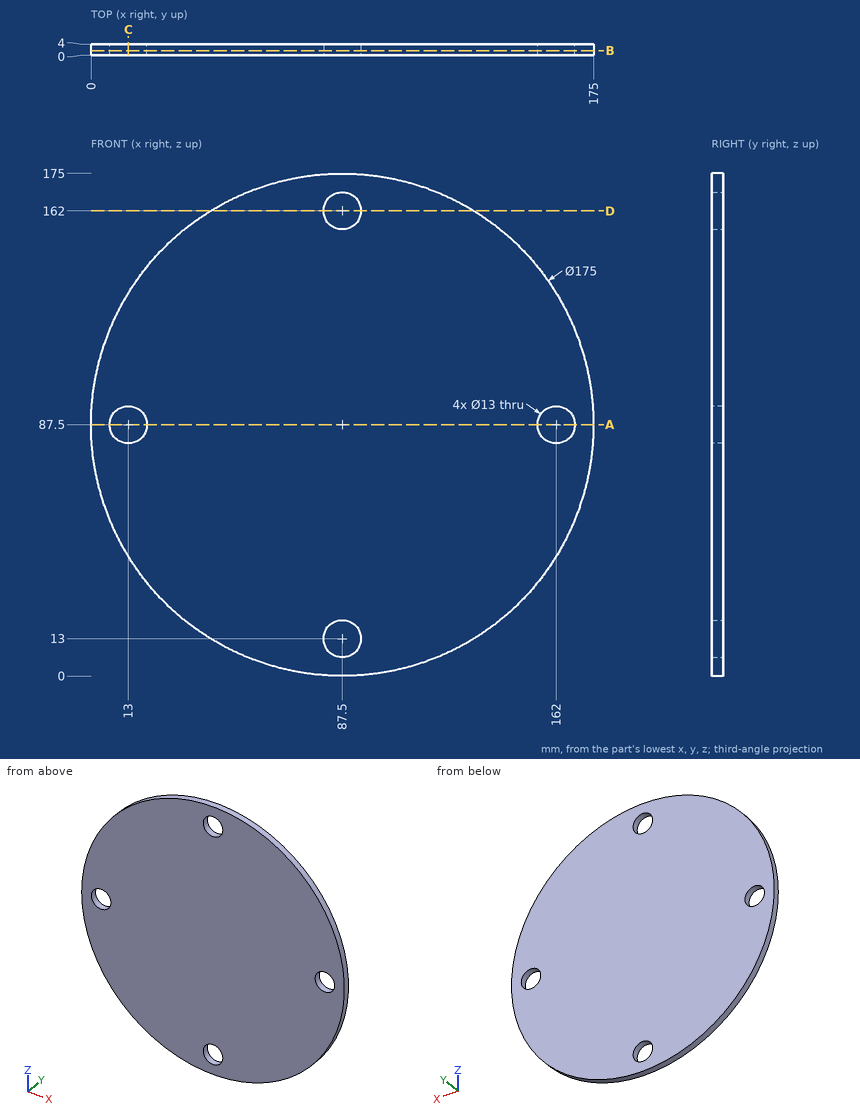
Part print with two shaded views. Sizes in mm from the minimum x, y, z corner. Coordinates: 2 decimals unless noted, no trailing zeros. Loops run counter-clockwise (first coordinate to the right, second up) from the corner with the lowest first, then second, coordinate; pieces in that order, holes last. Notation, with made-up numbers: (72.5, 43) - (86.5, 43) arc R32 ccw to (86.5, 71) - close; hole circle Ø10 at (38, -23). An arc over 180 degrees is marked (long way). Write each question's results on one line, items separated by ' | '. Start each with the question number.
Q1. Probe line 1 along Z through (x, y) = (87.5, 1.7); line 2 along Z through (x, y) = (86.5, 0.2); line 3 along X through (y, z) = (2.2, 7). List the from-to ranges inside material, lowest first.
Q2. Drop flat-ended pins along their axis: pin 1 Ø8 at (x, z) = (87.5, 13) entering from +Y; pin 2 Ø2 at (y, z) = (2, 131) entering from -X; pin 3 Ø1 at (y, z) = (1, 112) entering from +X; pin 4 Ø1.5 at (y, z) = (2.5, 37) entering from +X. Give the stop position or say it passes through.
Q3. Slice it at D-D on z = 162. Give the cut face in (x, y).
Q4. Slice it at C-C on x = 13. Give the cut face in (y, z), and give its area (3 significant figures).
Q5. Slice it at A-A on z = 87.5. Give the cut face in (x, y).
Q6. Slice it at B-B on y = 1.7. Give the cut face in (x, z).
Answer:
1) line 1: z = 0 to 6.5, 19.5 to 155.5, 168.5 to 175 | line 2: z = 0.01 to 6.58, 19.42 to 155.58, 168.42 to 174.99 | line 3: x = 53.21 to 85, 90 to 121.79
2) pin 1: passes through | pin 2: stops at x = 11.01 | pin 3: stops at x = 171.64 | pin 4: stops at x = 159.48
3) outline: (41.61, 0) - (81, 0) - (81, 4) - (41.61, 4) - close; (94, 0) - (133.39, 0) - (133.39, 4) - (94, 4) - close
4) outline: (0, 41.61) - (4, 41.61) - (4, 81) - (0, 81) - close; (0, 94) - (4, 94) - (4, 133.39) - (0, 133.39) - close | area: 315 mm2
5) outline: (0, 0) - (6.5, 0) - (6.5, 4) - (0, 4) - close; (19.5, 0) - (155.5, 0) - (155.5, 4) - (19.5, 4) - close; (168.5, 0) - (175, 0) - (175, 4) - (168.5, 4) - close
6) outline: circle Ø175 at (87.5, 87.5); hole circle Ø13 at (13, 87.5); hole circle Ø13 at (87.5, 13); hole circle Ø13 at (87.5, 162); hole circle Ø13 at (162, 87.5)
